Autodesk Inventor part; units mm, degrees
ref_plane "YZ Plane" through (0, 0, 0) normal (1, 0, 0) x (0, 1, 0)
ref_plane "XZ Plane" through (0, 0, 0) normal (0, 1, 0) x (-1, 0, 0)
ref_plane "XY Plane" through (0, 0, 0) normal (0, 0, 1) x (1, 0, 0)
sketch "Sketch1" plane through (0, 0, 0) normal (0, 0, 1) x (1, 0, 0)
  circle A0 centre (0, 0) radius 2.75
extrude "Extrusion3" add sketch "Sketch1" against normal blind 3
sketch "Sketch2" plane through (0, 0, 0) normal (0, 0, 1) x (1, 0, 0)
  circle A0 centre (0, 0) radius 1.5
extrude "Extrusion2" add sketch "Sketch2" along normal blind 14
sketch "Sketch3" plane through (0, 0, -3) normal (0, 0, -1) x (-1, 0, 0)
  line L0 (-0.7217, 1.25) -> (-1.4434, 0)
  line L1 (0.7217, -1.25) -> (1.4434, 0)
  line L2 (1.4434, 0) -> (0.7217, 1.25)
  line L3 (-1.4434, 0) -> (-0.7217, -1.25)
  line L4 (0.7217, 1.25) -> (-0.7217, 1.25)
  line L5 (-0.7217, -1.25) -> (0.7217, -1.25)
extrude "Extrusion1" cut sketch "Sketch3" against normal blind 3
fillet "Fillet2" radius 0.1 1 edges at (-2.75, 0, -3)
fillet "Fillet1" radius 0.1 1 edges at (-2.75, 0, 0)
chamfer "Chamfer1" distance 0.2 angle 45 1 edges at (-1.5, 0, 14)
properties part number "DIN 912 M3 12 mm"
For this review, take the finished solid that the model builds, in its own axes (mm). A direction names the side the tool comes from. Give positions to 0.01 mm unless a question says otherwise; leave off trailing zeros. Order: outer loops, then holes, each group sorted by start corner. A loop starts at its lowest first (then second) coordinate and runs counter-clockwise, first axis right, second up.
1) Insertion check: pin 1 (1.3 mm diameter, centred on x = -0.5, y = 0, fed in from -Z); pin 2 (2 mm diameter, centred on y = 2, z = 8.5, fed in from +X); pin 3 (2 mm diameter, centred on x = -0.5, z = 10, fed in from +Y). Each pin has a flat end and moves straight along its axis. Give the tip position at first contact, or say it passes through.
2) The part is to be moulded in two halves that separate along X. For faces 4 (the face through (-1.088, 0.616, -1.521)), 5 (the face through (0, -1.25, -2)), 6 (the face through (-0.596, -2.685, -1.48)), 7 (the face through (0, 0, 14)), say which applies: released by +X, released by -X, zero draft, split by the parting line, or undercut.
3) Take a section at A-A (x = 0). Give the boundary of the cut face in (y, z).
4) Wall thickness on line 1 (Z direction, x = -1.15, y = -1.8); line 2 (Y direction, x = 0.1, z = 3.5); line 3 (Y direction, x = -0.75, z = 1.25): over which ranges is each line inside the solid? List them lowest first.
5) Take a section at B-B (z = 5.25). Give the boundary of the cut face in (x, y), then the cut area to 3 significant figures.
6) For faces 1 (the face through (1.1, -1.1, -3)), 2 (the face through (0, -2, 0)), 3 (the face through (1.08, 0.63, -1.52)), list the 3-axis set-ups (+Z, -Z, +X, -X, +Y, -Y) from which the entire face can be reached by the end or side of a thin tool; tool diameter is ignored.
Derived:
1. pin 1: stops at z = 0
1. pin 2: stops at x = 1.12
1. pin 3: stops at y = 1.5
2. face 4: undercut
2. face 5: undercut
2. face 6: split by the parting line
2. face 7: zero draft
3. outline: (-2.75, -2.9) arc R0.1 ccw to (-2.65, -3) - (-1.25, -3) - (-1.25, 0) - (1.25, 0) - (1.25, -3) - (2.65, -3) arc R0.1 ccw to (2.75, -2.9) - (2.75, -0.1) arc R0.1 ccw to (2.65, 0) - (1.5, 0) - (1.5, 13.8) - (1.3, 14) - (-1.3, 14) - (-1.5, 13.8) - (-1.5, 0) - (-2.65, 0) arc R0.1 ccw to (-2.75, -0.1) - close
4. line 1: z = -3 to 0
4. line 2: y = -1.5 to 1.5
4. line 3: y = -1.3 to 1.3
5. outline: circle Ø3 at (0, 0)
5. area: 7.07 mm2
6. face 1: -Z, +X, -X, +Y, -Y
6. face 2: +Z
6. face 3: -Z
